Part model, mm, in its own coordinate system. Face numbers are marked on the shaded views. Round coordinates to 2 decimals unless told otherwise and drop trailing zeros. Write each loop counter-clockwise with the first axis right and the second up, starting at its lowest first coordinate (ties: lowest second). Pieces come first, ordered by that corner, then holes.
1) Saw through at C-C on z = 2.75. Write the cut outline in (x, y).
2) Saw through at B-B on x = 0. Write the cut outline in (y, z), and give its area (3 significant figures).
3) Drill centre lines: L1, parallel to Y at x = 0, z = 2.75; L2, parallel to X at y = -0.75, z = 4; L3, parallel to X at y = -0.25, z = 0.75. Where is each one in solid material? Low to high.
4) Saw through at A-A on y = 0. Write the cut outline in (x, z), and give its area (3 significant figures).
5) Pull direction X, two halves, no side cores. Call the marked faces 1, 2, 3 and 4: +X half, -X half, draft (parallel to the pull), parting line (faces both ways), or undercut.
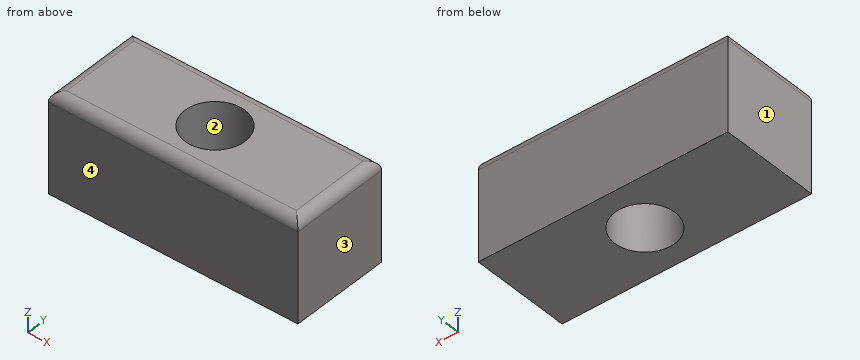
```python
from build123d import *

# Parameters (mm, degrees)
F0_W     = 25
F0_H     = 10
F1_DEPTH = 10
F3_R     = 1
F2_R     = 3
F2_R_2   = 1.5
F4_DEPTH = 10.001


with BuildPart() as f1:
    # F0 (on Top) → F1 (new body)
    with BuildSketch(Plane.XY):
        Rectangle(F0_W, F0_H)
    extrude(amount=F1_DEPTH)

    # F3
    f3_edges = [f1.edges().sort_by_distance(p)[0] for p in [
        (0, 5, 10),
        (12.5, 0, 10),
        (0, -5, 10),
        (-12.5, 0, 10),
    ]]
    fillet(f3_edges, radius=F3_R)

    # F2 (on face) → F4 (cut, through all)
    with BuildSketch(Plane.XY.offset(10)):
        Circle(F2_R)
        Circle(F2_R_2, mode=Mode.SUBTRACT)
        Circle(F2_R_2)
    extrude(amount=-F4_DEPTH, mode=Mode.SUBTRACT)


solid = f1.part
```
Completed:
1. outline: (-12.5, -5) - (12.5, -5) - (12.5, 5) - (-12.5, 5) - close; hole circle Ø6 at (0, 0)
2. outline: (-5, 0) - (-3, 0) - (-3, 10) - (-4, 10) arc R1 ccw to (-5, 9) - close; (3, 0) - (5, 0) - (5, 9) arc R1 ccw to (4, 10) - (3, 10) - close
2. area: 39.6 mm2
3. L1: y = -5 to -3, 3 to 5
3. L2: x = -12.5 to -2.9, 2.9 to 12.5
3. L3: x = -12.5 to -2.99, 2.99 to 12.5
4. outline: (-12.5, 0) - (-3, 0) - (-3, 10) - (-11.5, 10) arc R1 ccw to (-12.5, 9) - close; (3, 0) - (12.5, 0) - (12.5, 9) arc R1 ccw to (11.5, 10) - (3, 10) - close
4. area: 190 mm2
5. face 1: -X half
5. face 2: undercut
5. face 3: +X half
5. face 4: draft
